Verification items for the finished model (mm, model axes). Coordinates: 2 decimals unless noted, no trailing zeros. Order: outer loops, then holes, each group sorted by start corner. A loop starts at its lowest first (then second) coordinate and runs counter-clockwise, first axis right, second up. Notation, with made-up numbers: (56, -14.5) -> (63, -14.5) arc R5 cw to (63, -6.5) -> close; hole circle Ø7 at (46.5, 83.25). An arc over 180 degrees is marked (long way). Write each question's results on one line, items separated by ' | '. Start each with the question number.
(1) Cross-section at B-B on z = -0.55. Enter the section's corners in (x, y), and give its area (3 significant figures).
(2) Cross-section at C-C on y = 0. Enter the section's corners in (x, z).
(3) Draft check along X on faces 1 (the cylindrical face through (-1.84, -8.3, 0.02)), 2 (the flat face through (8, -3.3, -1.5)), 3 (the cylindrical face through (-1.951, 8.786, -0.021)). Enter one of: +X half, -X half, draft (parallel to the pull), parting line (faces both ways), or undercut.
(4) Cross-section at A-A on x = 0. Enter the section's corners in (y, z).
(5) Thickness scan on probe 1 along Z at (x, y) = (0, -8.65); probe 2 along X at (y, z) = (-7.75, -1.2); probe 3 along Y at (x, z) = (3.25, 0.95). Record the ranges inside material, lowest first. Write a range as [from, to].
(6) Go/stop test with flat-tipped pins: pin 1 (4 mm diameter, centred on x = 3.5, y = -6.5, fed in from +Z); pin 2 (1 mm diameter, centred on y = 5, z = 0.5, fed in from -X); pin 3 (1.5 mm diameter, centred on y = -2.5, z = 1, fed in from -X); pin 4 (1.5 mm diameter, centred on y = 2, z = 1, fed in from +X). Record where each tip stops, or that it passes through.
Autodesk Inventor part; units mm, degrees
ref_plane "Work Plane1" through (0, 9, 0) normal (0, 1, 0) x (-1, 0, 0)
ref_plane "YZ Plane" through (0, 0, 0) normal (1, 0, 0) x (0, 1, 0)
ref_plane "XY Plane" through (0, 0, 0) normal (0, 0, 1) x (1, 0, 0)
sketch "Sketch1" plane through (0, 0, 0) normal (0, 0, 1) x (1, 0, 0)
  circle A0 centre (0, 0) radius 9
  circle A1 centre (0, 0) radius 8.5
  dimension "d0" = 18
  dimension "d1" = 17
extrude "Extrusion1" add sketch "Sketch1" along normal mid plane 3
ref_plane "Work Plane1" through (0, 9, 0) normal (0, 1, 0) x (-1, 0, 0)
sketch "Sketch2" plane through (0, 9, 0) normal (0, 1, 0) x (-1, 0, 0)
  circle A0 centre (0, 0) radius 1.25
  dimension "d5" = 2.5
extrude "Extrusion2" cut sketch "Sketch2" against normal up to surface
mirror "Mirror1" about plane through (0, 0, 0) normal (0, 1, 0) of "Extrusion2"
properties part number "21.1"
Results are:
1) outline: (-1.12, -8.93) -> (-1.12, -8.43) arc R8.5 cw to (-1.12, 8.43) -> (-1.12, 8.93) arc R9 ccw to start; (1.12, -8.93) arc R9 ccw to (1.12, 8.93) -> (1.12, 8.43) arc R8.5 cw to (1.12, -8.43) -> close | area: 25.2 mm2
2) outline: (-9, -1.5) -> (-8.5, -1.5) -> (-8.5, 1.5) -> (-9, 1.5) -> close; (8.5, -1.5) -> (9, -1.5) -> (9, 1.5) -> (8.5, 1.5) -> close
3) face 1: undercut | face 2: draft | face 3: parting line
4) outline: (-9, -1.5) -> (-8.5, -1.5) -> (-8.5, -1.25) -> (-9, -1.25) -> close; (-9, 1.25) -> (-8.5, 1.25) -> (-8.5, 1.5) -> (-9, 1.5) -> close; (8.5, -1.5) -> (9, -1.5) -> (9, -1.25) -> (8.5, -1.25) -> close; (8.5, 1.25) -> (9, 1.25) -> (9, 1.5) -> (8.5, 1.5) -> close
5) probe 1: z = [-1.5, -1.25], [1.25, 1.5] | probe 2: x = [-4.58, -3.49], [3.49, 4.58] | probe 3: y = [-8.39, -7.85], [7.85, 8.39]
6) pin 1: stops at z = 1.5 | pin 2: stops at x = -7.79 | pin 3: stops at x = -8.83 | pin 4: stops at x = 8.91
